```python
from build123d import *

# Parameters (mm, degrees)
F1_DEPTH = 79.375


with BuildPart() as f1:
    # F0 (on Top) → F1 (new body)
    with BuildSketch(Plane.XY):
        Polygon((2.3622, 57.15), (-2.3622, 57.15), (-5.823357, 44.232787), (-12.509798, 55.814043), (-17.073218, 54.591279), (-17.073218, 41.218395), (-26.529275, 50.674452), (-30.620725, 48.312252), (-27.159568, 35.395039), (-38.740825, 42.08148), (-42.08148, 38.740825), (-35.395039, 27.159568), (-48.312252, 30.620725), (-50.674452, 26.529275), (-41.218395, 17.073218), (-54.591279, 17.073218), (-55.814043, 12.509798), (-44.232787, 5.823357), (-57.15, 2.3622), (-57.15, -2.3622), (-44.232787, -5.823357), (-55.814043, -12.509798), (-54.591279, -17.073218), (-41.218395, -17.073218), (-50.674452, -26.529275), (-48.312252, -30.620725), (-35.395039, -27.159568), (-42.08148, -38.740825), (-38.740825, -42.08148), (-27.159568, -35.395039), (-30.620725, -48.312252), (-26.529275, -50.674452), (-17.073218, -41.218395), (-17.073218, -54.591279), (-12.509798, -55.814043), (-5.823357, -44.232787), (-2.3622, -57.15), (2.3622, -57.15), (5.823357, -44.232787), (12.509798, -55.814043), (17.073218, -54.591279), (17.073218, -41.218395), (26.529275, -50.674452), (30.620725, -48.312252), (27.159568, -35.395039), (38.740825, -42.08148), (42.08148, -38.740825), (35.395039, -27.159568), (48.312252, -30.620725), (50.674452, -26.529275), (41.218395, -17.073218), (54.591279, -17.073218), (55.814043, -12.509798), (44.232787, -5.823357), (57.15, -2.3622), (57.15, 2.3622), (44.232787, 5.823357), (55.814043, 12.509798), (54.591279, 17.073218), (41.218395, 17.073218), (50.674452, 26.529275), (48.312252, 30.620725), (35.395039, 27.159568), (42.08148, 38.740825), (38.740825, 42.08148), (27.159568, 35.395039), (30.620725, 48.312252), (26.529275, 50.674452), (17.073218, 41.218395), (17.073218, 54.591279), (12.509798, 55.814043), (5.823357, 44.232787), align=None)
        with BuildLine():
            Line((-5, 33.575), (5, 33.575))
            Line((5, 33.575), (5, 28.134154))
            ThreePointArc((5, 28.134154), (0, -28.575), (-5, 28.134154))
            Line((-5, 28.134154), (-5, 33.575))
        make_face(mode=Mode.SUBTRACT)
    extrude(amount=F1_DEPTH)

    # F2 (on Front) → F3 (revolve, intersect)
    with BuildSketch(Plane.XZ):
        Polygon((0, -46.99), (0, 126.365), (-86.6775, 39.6875), align=None)
    revolve(axis=Axis((0, 0, 39.6875), (0, 0, -1)), mode=Mode.INTERSECT)


solid = f1.part
```
Check sheet for the modelled part. Datum: model origin and axes. Units: mm. Round coordinates to 2 decimals unless told otherwise and drop trailing zeros. Order: outer loops, then holes, each group sorted by start corner. A loop starts at its lowest first (then second) coordinate and runs counter-clockwise, first axis right, second up.
1) Section check B-B (y = 0). Record the boundary of the cut face in (x, z) (3 decimals), and give its area (3 significant figures).
2) Mould release check, pull along Y, two halves, no side actions. Record for faces 1 (the conical face through (49.313, -13.132, 75.333)), 2 (the flat face through (33.031, 38.785, 39.132)), 3 (the flat face through (-38.785, 33.031, 39.132)), 4 (the conical face through (-44.1, 25.4, 3.9)): +Y half, -Y half, draft (parallel to the pull), parting line (faces both ways), or undercut.
3) Scan lines: line 1 (X direction, y = 0, z = 45) (3 decimals); line 2 (X direction, y = 46, z = 33.5); line 3 (X direction, y = -41, z = 61.5). Record each from-to range of solid material in increasing order.
4) Go/stop test with flat-tipped pins: pin 1 Ø3 at (x, z) = (-26.5, 13.5) entering from +Y; pin 2 Ø6.5 at (y, z) = (50.5, 41.5) entering from -X; pin 3 Ø4 at (x, z) = (-44, 30) entering from -Y; pin 4 Ø12 at (x, y) = (-4, 34) entering from -Z. Record where each tip stops, or that it passes through.
5) Section check A-A (x = 0). Record the boundary of the cut face in (y, z) (3 decimals).
Result:
1. outline: (-57.15, 10.16) - (-46.99, 0) - (-28.575, 0) - (-28.575, 79.375) - (-46.99, 79.375) - (-57.15, 69.215) - close; (28.575, 0) - (46.99, 0) - (57.15, 10.16) - (57.15, 69.215) - (46.99, 79.375) - (28.575, 79.375) - close
1. area: 4,330 mm2
2. face 1: -Y half
2. face 2: undercut
2. face 3: undercut
2. face 4: +Y half
3. line 1: x = -57.15 to -28.575, 28.575 to 57.15
3. line 2: x = -30 to -21.85, -17.07 to -6.84, -5.35 to 5.35, 6.84 to 17.07, 21.85 to 30
3. line 3: x = -39.82 to -36.87, -28.66 to 28.66, 36.87 to 39.82
4. pin 1: stops at y = 50.67
4. pin 2: stops at x = -30.62
4. pin 3: stops at y = -38.82
4. pin 4: stops at z = 0
5. outline: (-57.15, 10.16) - (-46.99, 0) - (-28.575, 0) - (-28.575, 79.375) - (-46.99, 79.375) - (-57.15, 69.215) - close; (33.575, 0) - (46.99, 0) - (57.15, 10.16) - (57.15, 69.215) - (46.99, 79.375) - (33.575, 79.375) - close
